```python
from build123d import *

# Parameters (mm, degrees)
F0_W     = 44.45
F0_H     = 520.7
F1_DEPTH = 95.25
F0_W_2   = 774.7
F2_DEPTH = 25.4


with BuildPart() as f1:
    # F0 (on Top) → F1 (new body)
    with BuildSketch(Plane.XY):
        with Locations((408.446951, 2.281439)):
            Rectangle(F0_W, F0_H)
        Polygon((433.374935, -258.068561), (430.671951, -258.068561), (386.221951, -258.068561), (-388.478049, -258.068561), (-430.225065, -258.068561), (-430.225065, -302.518561), (433.374935, -302.518561), align=None)
        Polygon((-388.478049, 262.631439), (-432.928049, 262.631439), (-432.928049, -258.068561), (-430.225065, -258.068561), (-388.478049, -258.068561), align=None)
        Polygon((430.671951, 307.081439), (-432.928049, 307.081439), (-432.928049, 262.631439), (-388.478049, 262.631439), (386.221951, 262.631439), (430.671951, 262.631439), align=None)
    extrude(amount=F1_DEPTH)

    # F0 (on Top) → F2 (join)
    with BuildSketch(Plane.XY):
        with Locations((-1.128049, 2.281439)):
            Rectangle(F0_W_2, F0_H)
    extrude(amount=F2_DEPTH)


solid = f1.part
```
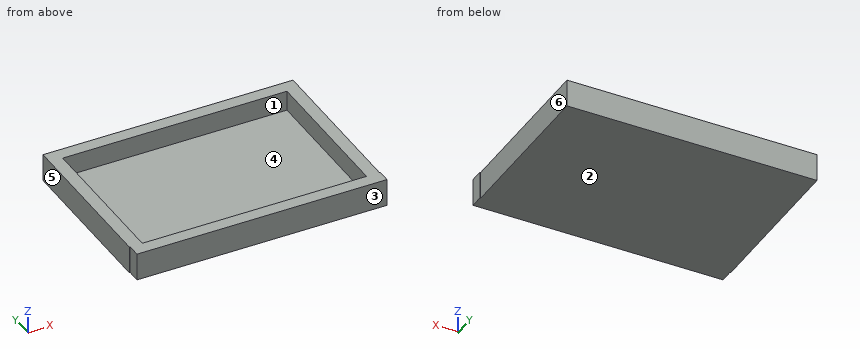
Model file for the job. Use its own axes, mm. Face numbers are marked on the shaded views. A direction names the side the tool comes from. Coordinates: 2 decimals unless noted, no trailing zeros. Loops run counter-clockwise (first coordinate to the right, second up) from the corner with the lowest first, then second, coordinate; pieces in that order, holes last. Notation, with made-up numbers: (-40, -3) - (-14, -3) arc R17 ccw to (-14, 18) - close; hole circle Ø1 at (-37.5, 61). An arc over 180 degrees is marked (long way). Answer as a JSON object with one key per item and string values. Group by question number.
(1) Cut at C-C (z = 72). Give the cut face in (x, y).
(2) Two-plate mould, pull along X, no slides. Class the marked faces 3, 4, 5 and 6: released by +X, released by -X, zero draft, split by the parting line, or undercut.
(3) Cut at B-B (y = -89.5). Give the cut face in (x, z).
(4) Flat gauge pins, fed straight in: pin 1 (4 mm diameter, centred on x = -317.5, y = 12.5, fed in from +Z); pin 2 (1.4 mm diameter, centred on x = 431.5, z = 50.5, fed in from +Y); pin 3 (2 mm diameter, centred on x = -431.5, z = 28.5, fed in from -Y). Where does each tip first touch, or does it go through?
(5) Probe line 1 along X through (y, z) = (64.5, 88); line 2 along Y through (x, z) = (363.5, 51.5); line 3 along Z through (x, y) = (-44, -8). List the from-to ranges inside material, lowest first.
(6) Tool access for the marked faces 1 and 2: list every direction of +Z, -Z, +X, -X, +Y, -Y with a clear straight run to the whole face (end or side of a thin tool).
(7) Cut at A-A (x = 248). Give the cut face in (y, z).
Geometry says:
{
 "1": {"outline": "(-432.93, -258.07) - (-430.23, -258.07) - (-430.23, -302.52) - (433.37, -302.52) - (433.37, -258.07) - (430.67, -258.07) - (430.67, 307.08) - (-432.93, 307.08) - close; hole (-388.48, -258.07) - (386.22, -258.07) - (386.22, 262.63) - (-388.48, 262.63) - close"},
 "2": {"face 3": "zero draft", "face 4": "undercut", "face 5": "released by -X", "face 6": "released by +X"},
 "3": {"outline": "(-432.93, 0) - (430.67, 0) - (430.67, 95.25) - (386.22, 95.25) - (386.22, 25.4) - (-388.48, 25.4) - (-388.48, 95.25) - (-432.93, 95.25) - close"},
 "4": {"pin 1": "stops at z = 25.4", "pin 2": "stops at y = -258.07", "pin 3": "stops at y = -258.07"},
 "5": {"line 1": "x = -432.93 to -388.48, 386.22 to 430.67", "line 2": "y = -302.52 to -258.07, 262.63 to 307.08", "line 3": "z = 0 to 25.4"},
 "6": {"face 1": "+Z", "face 2": "-Z, +X, -X, +Y, -Y"},
 "7": {"outline": "(-302.52, 0) - (307.08, 0) - (307.08, 95.25) - (262.63, 95.25) - (262.63, 25.4) - (-258.07, 25.4) - (-258.07, 95.25) - (-302.52, 95.25) - close"}
}
